Read the model definition and answer for the solid it produces. Units are mm, in the model's axes. Give positions to 0.01 mm unless a question says otherwise; leave off trailing zeros. Loops run counter-clockwise (first coordinate to the right, second up) from the corner with the lowest first, then second, coordinate; pieces in that order, holes last. Notation, with made-up numbers: (24.5, -2.5) - (65.5, -2.5) arc R25 cw to (65.5, 9.5) - close; hole circle Ø2 at (-10, 39.5). An arc over 180 degrees is marked (long way). Write item = value, one per line. Start each with the question number.
from build123d import *

# Parameters (mm, degrees)
SKETCH1_R           = 66.3575
BOSS_EXTRUDE1_DEPTH = 5.08
CUT_EXTRUDE2_REACH  = 95.981
SKETCH3_R           = 3.900616975
SKETCH3_W           = 5.08
SKETCH3_H           = 67.8815


with BuildPart() as part:
    # Sketch1 → Boss-Extrude1 (new body)
    with BuildSketch(Plane.XY):
        Circle(SKETCH1_R)
    extrude(amount=BOSS_EXTRUDE1_DEPTH)

    # Sketch3 → Cut-Extrude2 (cut, up to next)
    with BuildSketch(Plane.XY, mode=Mode.PRIVATE) as cut_extrude2_sk1:
        with BuildLine():
            Line((-50.832794134, -42.65377881), (-41.104029707, -34.490376167))
            ThreePointArc((-41.104029707, -34.490376167), (-50.4215568, -18.35194584), (-53.6575, 0))
            Line((-53.6575, 0), (-66.3575, 0))
            ThreePointArc((-66.3575, 0), (-62.355653084, -22.695601661), (-50.832794134, -42.65377881))
        make_face()
    cut_extrude2_tool1 = extrude(cut_extrude2_sk1.sketch, amount=CUT_EXTRUDE2_REACH, mode=Mode.PRIVATE) & part.part
    # Sketch3 → Cut-Extrude2 (cut, up to next)
    with BuildSketch(Plane.XY, mode=Mode.PRIVATE) as cut_extrude2_sk2:
        with BuildLine():
            ThreePointArc((50.832794134, 42.65377881), (62.355653084, 22.695601661), (66.3575, 0))
            Line((66.3575, 0), (53.6575, 0))
            ThreePointArc((53.6575, 0), (50.4215568, 18.35194584), (41.104029707, 34.490376167))
            Line((41.104029707, 34.490376167), (50.832794134, 42.65377881))
        make_face()
    cut_extrude2_tool2 = extrude(cut_extrude2_sk2.sketch, amount=CUT_EXTRUDE2_REACH, mode=Mode.PRIVATE) & part.part
    # Sketch3 → Cut-Extrude2 (cut, up to next)
    with BuildSketch(Plane.XY, mode=Mode.PRIVATE) as cut_extrude2_sk3:
        with Locations((15.41807752, -40.64)):
            Circle(SKETCH3_R)
    cut_extrude2_tool3 = extrude(cut_extrude2_sk3.sketch, amount=CUT_EXTRUDE2_REACH, mode=Mode.PRIVATE) & part.part
    # Sketch3 → Cut-Extrude2 (cut, up to next)
    with BuildSketch(Plane.XY, mode=Mode.PRIVATE) as cut_extrude2_sk4:
        with Locations((-15.06192248, -40.64)):
            Circle(SKETCH3_R)
    cut_extrude2_tool4 = extrude(cut_extrude2_sk4.sketch, amount=CUT_EXTRUDE2_REACH, mode=Mode.PRIVATE) & part.part
    # Sketch3 → Cut-Extrude2 (cut, up to next)
    with BuildSketch(Plane.XY, mode=Mode.PRIVATE) as cut_extrude2_sk5:
        with Locations(Location((15.41807752, 40.64, 0), (0, 0, 180))):
            Circle(SKETCH3_R)
    cut_extrude2_tool5 = extrude(cut_extrude2_sk5.sketch, amount=CUT_EXTRUDE2_REACH, mode=Mode.PRIVATE) & part.part
    # Sketch3 → Cut-Extrude2 (cut, up to next)
    with BuildSketch(Plane.XY, mode=Mode.PRIVATE) as cut_extrude2_sk6:
        with Locations(Location((-15.06192248, 40.64, 0), (0, 0, 180))):
            Circle(SKETCH3_R)
    cut_extrude2_tool6 = extrude(cut_extrude2_sk6.sketch, amount=CUT_EXTRUDE2_REACH, mode=Mode.PRIVATE) & part.part
    # Sketch3 → Cut-Extrude2 (cut, up to next)
    with BuildSketch(Plane.XY, mode=Mode.PRIVATE) as cut_extrude2_sk7:
        with Locations((0.17807752, -33.91789821)):
            Rectangle(SKETCH3_W, SKETCH3_H)
    cut_extrude2_tool7 = extrude(cut_extrude2_sk7.sketch, amount=CUT_EXTRUDE2_REACH, mode=Mode.PRIVATE) & part.part
    add(cut_extrude2_tool1.solids().sort_by_distance((-55.456661, -20.184574, 0))[0], mode=Mode.SUBTRACT)
    add(cut_extrude2_tool2.solids().sort_by_distance((55.456661, 20.184574, 0))[0], mode=Mode.SUBTRACT)
    add(cut_extrude2_tool3.solids().sort_by_distance((15.418078, -40.64, 0))[0], mode=Mode.SUBTRACT)
    add(cut_extrude2_tool4.solids().sort_by_distance((-15.061922, -40.64, 0))[0], mode=Mode.SUBTRACT)
    add(cut_extrude2_tool5.solids().sort_by_distance((15.418078, 40.64, 0))[0], mode=Mode.SUBTRACT)
    add(cut_extrude2_tool6.solids().sort_by_distance((-15.061922, 40.64, 0))[0], mode=Mode.SUBTRACT)
    add(cut_extrude2_tool7.solids().sort_by_distance((0.178078, -33.917898, 0))[0], mode=Mode.SUBTRACT)


solid = part.part
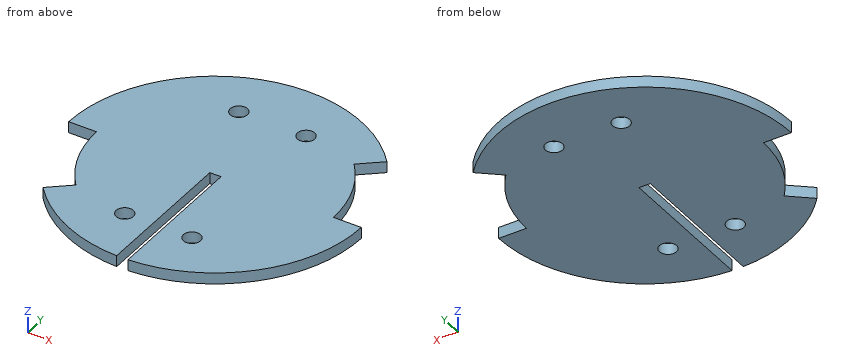
1. A cutting plane is placed at A-A on z = 1.45. Give the vertices of the cut face in (x, y) (1 decimal).
2. A cutting plane is placed at B-B on y = -3.5. Give the vertices of the cut face in (x, z).
3. A cutting plane is placed at D-D on x = -16. Give the vertices of the cut face in (y, z).
4. Consider line 1 along Y through (x, z) = (16, 2.5); line 2 along X through (y, z) = (40.64, 2.5); line 3 along X through (y, z) = (-52.5, 1.75). Determine where each line is inside the solid, lowest interval first. Write a range as [from, to].
5. A cutting plane is placed at C-C on y = 39. Give the vertices of the cut face in (x, z), and give its area (3 significant figures).
6. Given P1, Ø6, axis at x = 15.42, y = -40.64, coming from the -Z side; P2, Ø2.5, axis at y = -28.5, z = 3, coming from the +X side; P3, Ø1.5, axis at x = 3, z = 0.5, coming from the +Y side; P4, Ø1.5, axis at x = 59.5, z = 2.5, coming from the +Y side, each flat-ended and moving along its own axis, determine where each tip first touches the part or whether it passes through.
Reply:
q1.outline = (-66.4, 0) - (-53.7, 0) arc R53.7 ccw to (-41.1, -34.5) - (-50.8, -42.7) arc R66.4 ccw to (-2.4, -66.3) - (-2.4, 0) - (2.7, 0) - (2.7, -66.3) arc R66.4 ccw to (66.4, 0) - (53.7, 0) arc R53.7 ccw to (41.1, 34.5) - (50.8, 42.7) arc R66.4 ccw to start; hole circle Ø7.8 at (-15.1, -40.6); hole circle Ø7.8 at (-15.1, 40.6); hole circle Ø7.8 at (15.4, -40.6); hole circle Ø7.8 at (15.4, 40.6)
q2.outline = (-53.54, 0) - (-2.36, 0) - (-2.36, 5.08) - (-53.54, 5.08) - close; (2.72, 0) - (66.27, 0) - (66.27, 5.08) - (2.72, 5.08) - close
q3.outline = (-64.4, 0) - (-44.43, 0) - (-44.43, 5.08) - (-64.4, 5.08) - close; (-36.85, 0) - (36.85, 0) - (36.85, 5.08) - (-36.85, 5.08) - close; (44.43, 0) - (64.4, 0) - (64.4, 5.08) - (44.43, 5.08) - close
q4.line_1 = [-64.4, -44.5], [-36.78, 36.78], [44.5, 64.4]
q4.line_2 = [-52.46, -18.96], [-11.16, 11.52], [19.32, 48.43]
q4.line_3 = [-40.58, -2.36], [2.72, 40.58]
q5.outline = (-53.69, 0) - (-18.6, 0) - (-18.6, 5.08) - (-53.69, 5.08) - close; (-11.52, 0) - (11.88, 0) - (11.88, 5.08) - (-11.52, 5.08) - close; (18.96, 0) - (46.48, 0) - (46.48, 5.08) - (18.96, 5.08) - close
q5.area = 437 mm^2
q6.P1 = through
q6.P2 = 60.5
q6.P3 = 66.32
q6.P4 = 0
